Can you work these out from the drawing? Everything is in mm from the part's minimum corner. A direction names the side the tool comes from. Round coordinates to 2 decimals unless told otherwise and drop trailing zeros. Loops run counter-clockwise (first coordinate to the right, second up) from the corner with the lowest first, then second, coordinate; pieces in that order, holes last. Notation, with made-up numbers: (-40, 86.25) - (-26, 86.25) arc R34 cw to (-26, 122.25) - close; hole circle Ø2 at (34, 60). An arc over 180 degrees is marked (long way). Return JSON: item names as keys, results as strings. Group by question number.
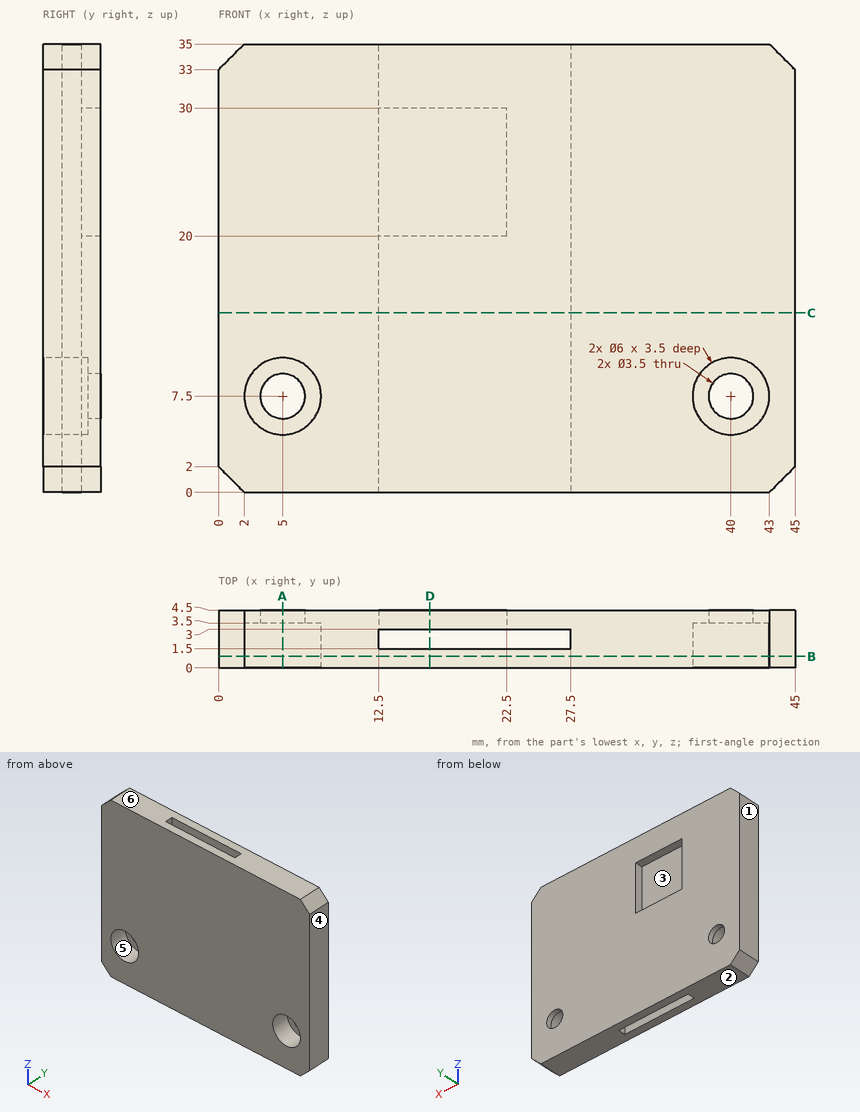
Q1. Imagine slicing it at B-B, the plane y = 0.9. List the corners of the cut face in (x, z) for me, and give its area (3 significant figures).
Q2. Imagine slicing it at C-C, the plane z = 14. List the corners of the cut face in (x, y) for me.
Q3. Imagine slicing it at D-D, the plane x = 16.5. List the corners of the cut face in (y, z) for me, and give its area (3 significant figures).
Q4. If we mould it in two halves opening along X, with no side actions, what happens to the marked faces 1, 2, 3 and 4? For each: +X half, -X half, draft (parallel to the pull), parting line (faces both ways), or undercut.
Q5. Please list where these lines run through material, in increasing order: line 1 (Z direction, x = 5, y = 4); line 2 (X direction, y = 2.35, z = 12.5); line 3 (Z direction, x = 40, y = 2.75).
Q6. Imagine slicing it at A-A, the plane x = 5. List the corners of the cut face in (y, z) for me, and give its area (3 significant figures).
Q7. For the marked faces 5 and 6, which set-ups out of +Z, -Z, +X, -X, +Y, -Y let a thin tool reach every point of the face, with its end or its side?
Q8. Will these pins go through, and if not, where does the flat tip stop? pin 1 Ø4.5 at (x, z) = (40, 7.5) entering from -Y; pin 2 Ø2 at (x, z) = (24, 27.5) entering from -Y.
Output values:
{
 "1": {"outline": "(0, 2) - (2, 0) - (43, 0) - (45, 2) - (45, 33) - (43, 35) - (2, 35) - (0, 33) - close; hole circle Ø6 at (5, 7.5); hole circle Ø6 at (40, 7.5)", "area": "1,510 mm^2"},
 "2": {"outline": "(0, 0) - (45, 0) - (45, 4.5) - (0, 4.5) - close; hole (12.5, 1.5) - (27.5, 1.5) - (27.5, 3) - (12.5, 3) - close"},
 "3": {"outline": "(0, 0) - (1.5, 0) - (1.5, 35) - (0, 35) - close; (3, 0) - (4.5, 0) - (4.5, 20) - (3, 20) - close; (3, 30) - (4.5, 30) - (4.5, 35) - (3, 35) - close", "area": "90.0 mm^2"},
 "4": {"face 1": "-X half", "face 2": "draft", "face 3": "undercut", "face 4": "+X half"},
 "5": {"line 1": "z = 0 to 5.75, 9.25 to 35", "line 2": "x = 0 to 12.5, 27.5 to 45", "line 3": "z = 0 to 4.5, 10.5 to 35"},
 "6": {"outline": "(0, 0) - (4.5, 0) - (4.5, 5.75) - (3.5, 5.75) - (3.5, 4.5) - (0, 4.5) - close; (0, 10.5) - (3.5, 10.5) - (3.5, 9.25) - (4.5, 9.25) - (4.5, 35) - (0, 35) - close", "area": "133 mm^2"},
 "7": {"face 5": "-Y", "face 6": "+Z, +X, -X, +Y, -Y"},
 "8": {"pin 1": "stops at y = 3.5", "pin 2": "stops at y = 0"}
}
